Part print with two shaded views. Sizes in mm from the minimum x, y, z corner. Give positions to 0.01 mm unless a question says otherwise; leave off trailing zeros. Write each loop counter-clockwise with the first axis right and the second up, starting at its lowest first coordinate (ties: lowest second). Pieces come first, ordered by that corner, then holes.
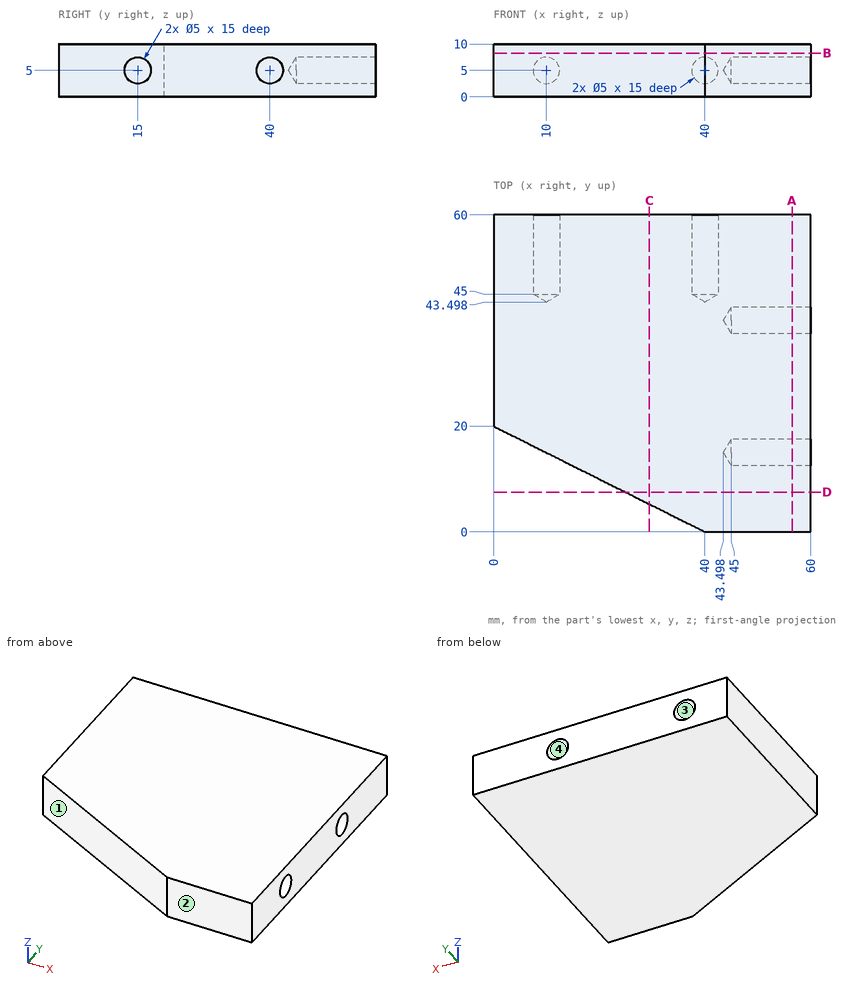
1) Flat gauge pins, fed straight in: P1, Ø5, axis at y = 12, z = 3.5, coming from the -X side; P2, Ø4.5, axis at y = 15, z = 5, coming from the -X side; P3, Ø3, axis at x = 10, z = 5, coming from the -Y side. Where does each tip first touch, or does it go through?
Check result:
P1: stops at x = 11
P2: stops at x = 5.5
P3: stops at y = 14.25
2) Saw through at A-A (x = 56.5). Write the cut outline in (y, z).
Check result:
outline: (0, 0) - (60, 0) - (60, 10) - (0, 10) - close; hole circle Ø5 at (15, 5); hole circle Ø5 at (40, 5)
3) Mould opens along X. For the marked faces 1, 2, 3 and 4 say: +X half, -X half, draft (parallel to the pull), parting line (faces both ways), or undercut.
Check result:
face 1: -X half
face 2: draft
face 3: undercut
face 4: undercut
4) Drill centre lines: L1, parallel to Y at x = 46, z = 4.75; L2, parallel to Y at x = 57, z = 3.25 (1 decimal); L3, parallel to Z at x = 10, y = 49. Where is each one in solid material? Low to high.
Check result:
L1: y = 0 to 12.51, 17.49 to 37.51, 42.49 to 60
L2: y = 0 to 13.2, 16.8 to 38.2, 41.8 to 60
L3: z = 0 to 2.5, 7.5 to 10
5) Saw through at C-C (x = 29.5). Write the cut outline in (y, z).
Check result:
outline: (5.25, 0) - (60, 0) - (60, 10) - (5.25, 10) - close
6) Saw through at B-B (z = 8.25). Write the cut outline in (x, y), and give its area (3 significant figures).
Check result:
outline: (0, 20) - (40, 0) - (60, 0) - (60, 60) - (0, 60) - close
area: 3,200 mm2
7) Saw through at D-D (y = 7.5). Write the cut outline in (x, z), and give its area (3 significant figures).
Check result:
outline: (25, 0) - (60, 0) - (60, 10) - (25, 10) - close
area: 350 mm2
